Build history of the part. All positions in model axes, mm. A direction names the side the tool comes from. Round coordinates to 2 decimals unless told otherwise and drop trailing zeros. Loops run counter-clockwise (first coordinate to the right, second up) from the corner with the lowest first, then second, coordinate; pieces in that order, holes last. Notation, with made-up numbers: (8, -39) -> (46, -39) arc R14 ccw to (46, -35) -> close; hole circle Ø10 at (28, 64.25). An arc over 180 degrees is marked (long way). Put each result on its own line as item: value. Start each with the question number.
Item 1: Flat gauge pins, fed straight in: pin 1 Ø1.5 at (y, z) = (9, -5) entering from -X; pin 2 Ø4 at (x, y) = (-8.5, 30.5) entering from -Z; pin 3 Ø4 at (x, z) = (0.5, -4) entering from +Y. Where does each tip first touch, or does it go through?
Item 2: Drill centre lines: probe 1 along X at (y, z) = (7.5, 0); probe 2 along Z at (x, y) = (0.5, 21.5). Where is each one in solid material? Low to high. Write a range as [from, to].
Item 3: Tool access for faces 1 (the cylindrical face through (-13.31, 35.21, 6.92)), 2 (the cylindrical face through (10.4, 24.99, -3.27)): list every direction of +Z, -Z, +X, -X, +Y, -Y with a clear straight run to the whole face (end or side of a thin tool).
Item 4: Cut at B-B, the plane y = 8.5. List the corners of the cut face in (x, z), plus the area to 3 significant figures.
Item 5: Cut at A-A, the plane y = 22. List the corners of the cut face in (x, z).
```python
from build123d import *

# Parameters (mm, degrees)
SKETCH1_R           = 8
BOSS_EXTRUDE1_DEPTH = 20.5
SKETCH2_R           = 10.3
BOSS_EXTRUDE2_DEPTH = 4
SKETCH3_R           = 10.9
BOSS_EXTRUDE3_DEPTH = 1
SKETCH4_R           = 12.8
BOSS_EXTRUDE4_DEPTH = 6.5
FILLET1_R           = 2


with BuildPart() as part:
    # Sketch1 → Boss-Extrude1 (new body)
    with BuildSketch(Plane(origin=(0, 0, 0), x_dir=(1, 0, 0), z_dir=(0, 1, 0))):
        Circle(SKETCH1_R)
    extrude(amount=BOSS_EXTRUDE1_DEPTH)

    # Sketch2 → Boss-Extrude2 (add)
    with BuildSketch(Plane(origin=(0, 20.5, 0), x_dir=(1, 0, 0), z_dir=(0, 1, 0))):
        Circle(SKETCH2_R)
    extrude(amount=BOSS_EXTRUDE2_DEPTH)

    # Sketch3 → Boss-Extrude3 (add)
    with BuildSketch(Plane(origin=(0, 24.5, 0), x_dir=(1, 0, 0), z_dir=(0, 1, 0))):
        Circle(SKETCH3_R)
    extrude(amount=BOSS_EXTRUDE3_DEPTH)

    # Sketch4 → Boss-Extrude4 (add)
    with BuildSketch(Plane(origin=(0, 25.5, 0), x_dir=(1, 0, 0), z_dir=(0, 1, 0))):
        Circle(SKETCH4_R)
    extrude(amount=BOSS_EXTRUDE4_DEPTH)

    # Sketch5 → Revolve1 (revolve)
    with BuildSketch(Plane(origin=(0, 0, 0), x_dir=(0, 0, -1), z_dir=(1, 0, 0))):
        with BuildLine():
            Line((0, 32), (0, 40))
            ThreePointArc((0, 40), (-7.566372975, 39.497797314), (-15, 38))
            Line((-15, 38), (-15, 32))
            Line((-15, 32), (-12.8, 32))
            Line((-12.8, 32), (0, 32))
        make_face()
    revolve(axis=Axis((0, 32, 0), (0, 1, 0)))

    # Fillet1
    fillet1_edges = [part.edges().sort_by_distance(p)[0] for p in [
        (0, 38, -15),
        (0, 32, -15),
    ]]
    fillet(fillet1_edges, radius=FILLET1_R)


solid = part.part
```
Reply:
1. pin 1: stops at x = -6.78
1. pin 2: stops at z = -11.82
1. pin 3: stops at y = 39.96
2. probe 1: x = [-8, 8]
2. probe 2: z = [-10.29, 10.29]
3. face 1: +Y, -Y
3. face 2: -Y
4. outline: circle Ø16 at (0, 0)
4. area: 201 mm^2
5. outline: circle Ø20.6 at (0, 0)
